Here's how the part is built. I have some questions about the finished solid (model axes, mm). Give positions to 0.01 mm unless a question says otherwise; leave off trailing zeros. Order: outer loops, then holes, each group sorted by start corner. A loop starts at its lowest first (then second) coordinate and runs counter-clockwise, first axis right, second up.
from build123d import *

# Parameters (mm, degrees)
SKETCH1_R           = 11
SKETCH1_R_2         = 3
SKETCH1_R_3         = 1.5
BOSS_EXTRUDE1_DEPTH = 2
SKETCH2_R           = 5
SKETCH2_R_2         = 3
BOSS_EXTRUDE2_DEPTH = 10
CHAMFER1_SIZE       = 0.5
CHAMFER2_SIZE       = 0.1
CUT_EXTRUDE1_DEPTH  = 10


with BuildPart() as part:
    # Sketch1 → Boss-Extrude1 (new body)
    with BuildSketch(Plane(origin=(0, 0, 0), x_dir=(1, 0, 0), z_dir=(0, 1, 0))):
        Circle(SKETCH1_R)
        Circle(SKETCH1_R_2, mode=Mode.SUBTRACT)
        with Locations((0, 8)):
            Circle(SKETCH1_R_3, mode=Mode.SUBTRACT)
        with Locations((8, 0)):
            Circle(SKETCH1_R_3, mode=Mode.SUBTRACT)
        with Locations((0, -8)):
            Circle(SKETCH1_R_3, mode=Mode.SUBTRACT)
        with Locations((-8, 0)):
            Circle(SKETCH1_R_3, mode=Mode.SUBTRACT)
    extrude(amount=BOSS_EXTRUDE1_DEPTH)

    # Sketch2 → Boss-Extrude2 (add)
    with BuildSketch(Plane(origin=(0, 2, 0), x_dir=(1, 0, 0), z_dir=(0, 1, 0))):
        Circle(SKETCH2_R)
        Circle(SKETCH2_R_2, mode=Mode.SUBTRACT)
    extrude(amount=BOSS_EXTRUDE2_DEPTH)

    # Chamfer1
    chamfer1_edges = [part.edges().sort_by_distance(p)[0] for p in [
        (-5, 12, 0),
    ]]
    chamfer(chamfer1_edges, length=CHAMFER1_SIZE)

    # Chamfer2
    chamfer2_edges = [part.edges().sort_by_distance(p)[0] for p in [
        (-1.5, 2, -8),
        (-1.5, 2, 8),
        (-5, 2, 0),
        (-9.5, 2, 0),
        (6.5, 2, 0),
        (-11, 2, 0),
        (-11, 0, 0),
    ]]
    chamfer(chamfer2_edges, length=CHAMFER2_SIZE)

    # Sketch3 → Cut-Extrude1 (cut)
    with BuildSketch(Plane.XY.offset(5)):
        with BuildLine():
            ThreePointArc((0, 10), (-1.5, 8.5), (0, 7))
            Line((0, 7), (0, 10))
        make_face()
        with BuildLine():
            Line((0, 10), (0, 7))
            ThreePointArc((0, 7), (1.060660172, 7.439339828), (1.5, 8.5))
            ThreePointArc((1.5, 8.5), (1.060660172, 9.560660172), (0, 10))
        make_face()
    extrude(amount=-CUT_EXTRUDE1_DEPTH, mode=Mode.SUBTRACT)


solid = part.part
Q1. I need wall thicknesses on L1, parallel to X at y = 1.25, z = 0; L2, parallel to X at y = 7.5, z = 0. Which ranges of each line are inside material? Lowest first, please.
Filled sheet:
L1: x = -11 to -9.5, -6.5 to -3, 3 to 6.5, 9.5 to 11
L2: x = -5 to -3, 3 to 5
Q2. If we section it at B-B on y = 7.5: List the corners of the cut face in (x, z) for me.
Filled sheet:
outline: (-1.12, -4.87) - (-1.12, -2.78) arc R3 cw to (-1.12, 2.78) - (-1.12, 4.87) arc R5 ccw to start; (1.12, -4.87) arc R5 ccw to (1.12, 4.87) - (1.12, 2.78) arc R3 cw to (1.12, -2.78) - close
Q3. Thinking about a two-plate mould opening in Z: for faces 1 (the face through (5, 2, 2)), 2 (the face through (2.77, 5.92, 1.15)), 3 (the face through (4.77, 6.73, -1.5)), which applies, released by +Z, released by -Z, zero draft, split by the parting line, or undercut?
Filled sheet:
face 1: zero draft
face 2: undercut
face 3: split by the parting line
Q4. I'm going to push flat-ended pins straight in: P1, Ø5, axis at x = 8, z = 2.5, coming from the +Y side; P2, Ø2.5, axis at x = 8, z = 0, coming from the +Y side; P3, Ø1, axis at y = 11, z = -1, coming from the -X side. Where does each tip first touch, or does it pass through?
Filled sheet:
P1: stops at y = 2
P2: passes through
P3: stops at x = -4.97
Q5. If we section it at C-C on y = 5.75: List the corners of the cut face in (x, z) for me, plus the area to 3 significant figures.
Filled sheet:
outline: circle Ø10 at (0, 0); hole circle Ø6 at (0, 0)
area: 50.3 mm2
Q6. If we section it at A-A on z = 0: Give the number of separate pieces and of enclosed holes in the cut face, plus the area to 3 significant figures.
Filled sheet:
separate pieces: 4
enclosed holes: 0
area: 59.7 mm2
